Geometry: final body of the model. Coordinates: model frame, mm. Round coordinates to 2 decimals unless told otherwise and drop trailing zeros. Loops run counter-clockwise (first coordinate to the right, second up) from the corner with the lowest first, then second, coordinate; pieces in that order, holes last. Notation, with made-up numbers: (13.5, 78) -> (19.5, 78) arc R17 ccw to (19.5, 109) -> close; hole circle Ø7 at (-32.5, 45). An arc over 180 degrees is marked (long way). Answer in a Markdown table with one row per item.
```python
from build123d import *

# Parameters (mm, degrees)
BOSS_EXTRUDE2_DEPTH = 4
SKETCH10_R          = 0.6
CUT_EXTRUDE3_DEPTH  = 2
SKETCH14_R          = 0.6
CUT_EXTRUDE5_DEPTH  = 2.6
SKETCH15_R          = 0.6
CUT_EXTRUDE6_DEPTH  = 3
FILLET3_R           = 0.2


with BuildPart() as part:
    # Sketch3 → Boss-Extrude2 (new body)
    with BuildSketch(Plane(origin=(0, 0, 0), x_dir=(0, 0, -1), z_dir=(1, 0, 0))):
        Polygon((-20.123053839, -5.770870406), (-14.550172907, -5.770870406), (-13.712271186, -8.337564915), (-13.712271186, -9.037564915), (-15.212271186, -9.037564915), (-15.212271186, -8.537564915), (-19.46095556, -8.537564915), (-19.46095556, -9.037564915), (-20.96095556, -9.037564915), (-20.96095556, -8.337564915), align=None)
    extrude(amount=BOSS_EXTRUDE2_DEPTH)

    # Sketch5 → Revolve2 (revolve)
    with BuildSketch(Plane(origin=(2, 0, 0), x_dir=(0, 0, -1), z_dir=(1, 0, 0)), mode=Mode.PRIVATE) as revolve2_sk:
        Polygon((-19.841868378, -5.839481614), (-19.511618443, -5.839481614), (-19.511618443, -3.21350004), (-19.841868378, -3.21350004), (-19.841868378, -3.686663005), (-20.121551797, -4.10664197), (-20.121551797, -4.205331029), (-19.841868378, -4.205331029), (-19.841868378, -4.519502648), (-20.121551797, -4.939481613), (-20.121551797, -5.036674624), (-19.841868378, -5.036674624), align=None)
    revolve(revolve2_sk.sketch.rotate(Axis((2, -5.639481613, 18.911618443), (0, 1, 0)), 180), axis=Axis((2, -5.639481613, 18.911618443), (0, 1, 0)))

    # Sketch6 → Revolve3 (revolve)
    with BuildSketch(Plane(origin=(2, 0, 0), x_dir=(0, 0, -1), z_dir=(1, 0, 0)), mode=Mode.PRIVATE) as revolve3_sk:
        Polygon((-16.605788013, -6.065180205), (-16.275538078, -6.065180205), (-16.275538078, -3.44200562), (-16.605788013, -3.44200562), (-16.605788013, -3.915168585), (-16.885471432, -4.335147551), (-16.885471432, -4.433836609), (-16.605788013, -4.433836609), (-16.605788013, -4.748008228), (-16.885471432, -5.167987194), (-16.885471432, -5.265180205), (-16.605788013, -5.265180205), align=None)
    revolve(revolve3_sk.sketch.rotate(Axis((2, -6.067987194, 15.675538078), (0, 1, 0)), 180), axis=Axis((2, -6.067987194, 15.675538078), (0, 1, 0)))

    # Sketch10 → Cut-Extrude3 (cut)
    with BuildSketch(Plane(origin=(0, -5.770870406, 0), x_dir=(1, 0, 0), z_dir=(0, 1, 0))):
        with Locations(Location((2, -18.911618443, 0), (0, 0, 90))):
            Circle(SKETCH10_R)
        with Locations(Location((2, -15.675538078, 0), (0, 0, 90))):
            Circle(SKETCH10_R)
    extrude(amount=-CUT_EXTRUDE3_DEPTH, mode=Mode.SUBTRACT)

    # Sketch12 → Revolve5 (revolve)
    with BuildSketch(Plane(origin=(0, -7, 0), x_dir=(1, 0, 0), z_dir=(0, 1, 0)), mode=Mode.PRIVATE) as revolve5_sk:
        Polygon((0, -16.405788013), (0, -16.075538078), (-2.425981573, -16.075538078), (-2.425981573, -16.405788013), (-1.952818609, -16.405788013), (-1.532839643, -16.685471432), (-1.434150585, -16.685471432), (-1.434150585, -16.405788013), (-1.119978965, -16.405788013), (-0.7, -16.685471432), (-0.602806989, -16.685471432), (-0.602806989, -16.405788013), align=None)
    revolve(revolve5_sk.sketch.rotate(Axis((0, -7, 15.475538078), (-1, 0, 0)), 180), axis=Axis((0, -7, 15.475538078), (-1, 0, 0)))

    # Sketch13 → Revolve6 (revolve)
    with BuildSketch(Plane(origin=(0, -7, 0), x_dir=(1, 0, 0), z_dir=(0, 1, 0))):
        Polygon((4.553932823, -20.292068689), (4.553932823, -20.012385269), (3.951125834, -20.012385269), (3.951125834, -19.682135334), (6.377107408, -19.682135334), (6.377107408, -20.012385269), (5.903944443, -20.012385269), (5.483965478, -20.292068689), (5.385276419, -20.292068689), (5.385276419, -20.012385269), (5.0711048, -20.012385269), (4.651125834, -20.292068689), align=None)
    revolve(axis=Axis((3.951125834, -7, 19.082135334), (1, 0, 0)))

    # Sketch14 → Cut-Extrude5 (cut)
    with BuildSketch(Plane.ZY):
        with Locations(Location((15.475538078, -7, 0), (0, 0, 180))):
            Circle(SKETCH14_R)
    extrude(amount=-CUT_EXTRUDE5_DEPTH, mode=Mode.SUBTRACT)

    # Sketch15 → Cut-Extrude6 (cut)
    with BuildSketch(Plane(origin=(4, 0, 0), x_dir=(0, 0, -1), z_dir=(1, 0, 0))):
        with Locations(Location((-19.082135334, -7, 0), (0, 0, 180))):
            Circle(SKETCH15_R)
    extrude(amount=-CUT_EXTRUDE6_DEPTH, mode=Mode.SUBTRACT)

    # Fillet3
    fillet3_edges = [part.edges().sort_by_distance(p)[0] for p in [
        (2, -3.21350004, 19.841868378),
        (2, -3.44200562, 16.605788013),
        (-2.425981573, -7, 16.405788013),
    ]]
    fillet(fillet3_edges, radius=FILLET3_R)


solid = part.part
```
Item 1: Line query: probe 1 along Z at (x, y) = (-1.3, -7); probe 2 along X at (y, z) = (-6.5, 20); probe 3 along Z at (x, y) = (2.75, -8.65). Output: solid intervals per line, ascending. Write a range as [from, to].
Answer:
| item | result |
|---|---|
| probe 1 | z = [14.55, 14.88], [16.08, 16.41] |
| probe 2 | x = [0, 4], [4.55, 4.9], [5.39, 5.73] |
| probe 3 | z = [13.71, 15.21], [19.46, 20.96] |
Item 2: Pin query (flat end, axial travel): pin 1 Ø1.2 at (y, z) = (-7.5, 19.5) entering from -X; pin 2 Ø1.5 at (y, z) = (-8.5, 18) entering from +X; pin 3 Ø1 at (y, z) = (-6.5, 16.5) entering from -X; pin 4 Ø0.7 at (x, z) = (2, 19) entering from -Y. Return the tip coordinate at first contact, or that it passes through.
Answer:
| item | result |
|---|---|
| pin 1 | stops at x = 0 |
| pin 2 | stops at x = 5.65 |
| pin 3 | stops at x = -2.43 |
| pin 4 | stops at y = -8.54 |
Item 3: Draft query along Y for faces 1 (the face through (2, -9.038, 14)), 2 (the face through (6.14, -7.28, 19.97)), 3 (the face through (1.2, -5.5, 15.2)). Return one class per face: pulls with the +Y half, pulls with the -Y half, needs draft (parallel to the pull), parting line crosses it, or undercut.
Answer:
| item | result |
|---|---|
| face 1 | pulls with the -Y half |
| face 2 | parting line crosses it |
| face 3 | undercut |
Item 4: Cut plane B-B (z = 20.5). Output: boundary loops of the cut face in (x, y).
Answer:
| item | result |
|---|---|
| outline | (0, -9.04) -> (4, -9.04) -> (4, -6.93) -> (0, -6.93) -> close |
Item 5: Cut plane A-A (z = 17). Output: boundary loops of the cut face in (x, y), then the cut area to 3 significant figures.
Answer:
| item | result |
|---|---|
| outline | (0, -8.54) -> (4, -8.54) -> (4, -5.77) -> (0, -5.77) -> close |
| area | 11.1 mm² |
